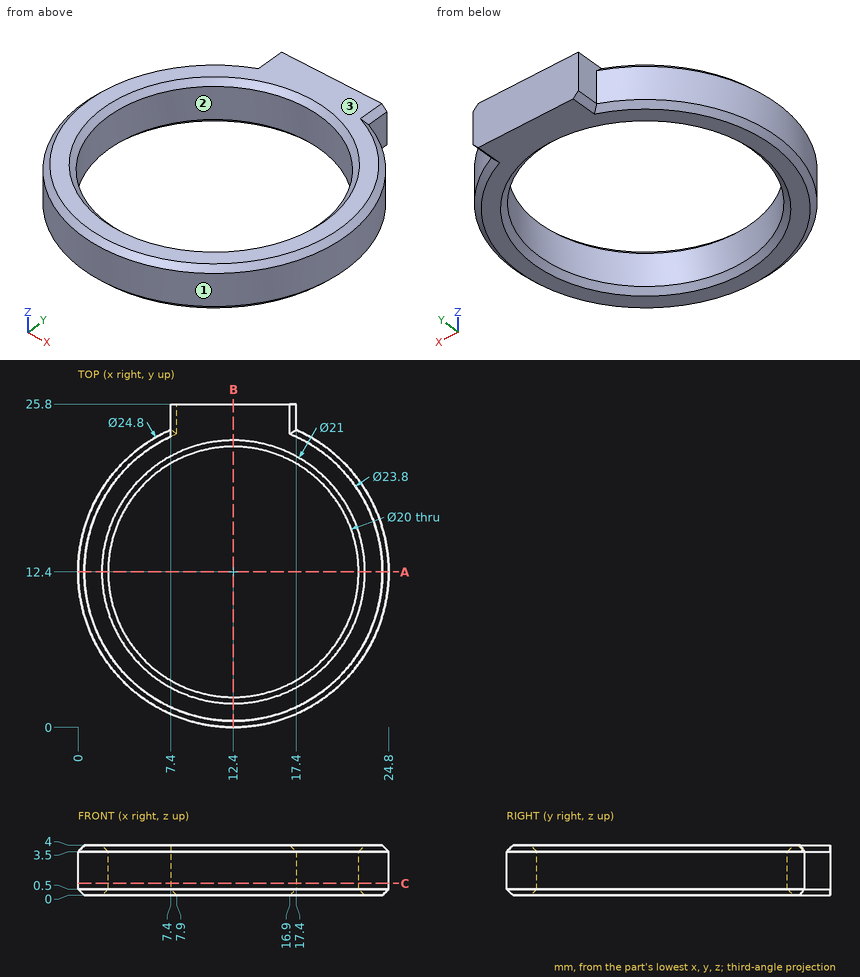
Could you check a few things on this drawing? It's one solid part, dimensions in mm from its lowest x, y, z. Coordinates: 2 decimals unless noted, no trailing zeros. Write each loop counter-clockwise with the first axis right and the second up, starting at its lowest first coordinate (ties: lowest second). Pieces come first, ordered by that corner, then holes. Notation, with made-up numbers: (26.5, 32) - (30.5, 32) arc R10 cw to (30.5, 42) - close; hole circle Ø8 at (48, 26). An arc over 180 degrees is marked (long way). Return JSON: item names as keys, results as strings. Group by question number.
Item 1: If we section it at A-A (y = 12.4): Write out the boundary of the cut face in (x, z).
Item 2: Please list where these lines run through material, in increasing order: probe 1 along Y at (x, z) = (12.4, 2.8); probe 2 along Y at (x, z) = (6, 1.25); probe 3 along X at (y, z) = (8.25, 2.2).
Item 3: If we section it at C-C (z = 0.95): Write out the boundary of the cut face in (x, y), then the cut area to 3 significant figures.
Item 4: We'd pull the mould along X, two halves only. Please class the marked faces 1, 2 and 3: pulls with the +X half, pulls with the -X half, needs draft (parallel to the pull), parting line crosses it, or undercut.
Item 5: If we section it at B-B (x = 12.4): Write out the boundary of the cut face in (y, z), then the cut area to 4 significant figures.
Item 6: I'm going to push flat-ended pins straight in: pin 1 Ø1.5 at (x, z) = (3, 3.5) entering from -Y; pin 2 Ø1 at (y, z) = (24.5, 2.5) entering from +X; pin 3 Ø0.8 at (y, z) = (25, 2) entering from -X. Where does each tip first touch, or does it pass through?
Return value:
{
 "1": {"outline": "(0, 0.5) - (0.5, 0) - (1.9, 0) - (2.4, 0.5) - (2.4, 3.5) - (1.9, 4) - (0.5, 4) - (0, 3.5) - close; (22.4, 0.5) - (22.9, 0) - (24.3, 0) - (24.8, 0.5) - (24.8, 3.5) - (24.3, 4) - (22.9, 4) - (22.4, 3.5) - close"},
 "2": {"probe 1": "y = 0 to 2.4, 22.4 to 25.8", "probe 2": "y = 1.78 to 4.72, 20.08 to 23.02", "probe 3": "x = 0.72 to 3.3, 21.5 to 24.08"},
 "3": {"outline": "(7.4, 23.75) arc R12.4 ccw (long way) to (17.4, 23.75) - (17.4, 25.8) - (7.4, 25.8) - close; hole circle Ø20 at (12.4, 12.4)", "area": "182 mm^2"},
 "4": {"face 1": "parting line crosses it", "face 2": "undercut", "face 3": "needs draft"},
 "5": {"outline": "(0, 0.5) - (0.5, 0) - (1.9, 0) - (2.4, 0.5) - (2.4, 3.5) - (1.9, 4) - (0.5, 4) - (0, 3.5) - close; (22.4, 0.5) - (22.9, 0) - (25.8, 0) - (25.8, 4) - (22.9, 4) - (22.4, 3.5) - close", "area": "22.45 mm^2"},
 "6": {"pin 1": "stops at y = 3.52", "pin 2": "stops at x = 17.4", "pin 3": "stops at x = 7.4"}
}
